The model under review builds one solid part; all positions refer to its coordinate system, in mm. A direction names the side the tool comes from. Round coordinates to 2 decimals unless told otherwise and drop trailing zeros. Loops run counter-clockwise (first coordinate to the right, second up) from the corner with the lowest first, then second, coordinate; pieces in that order, holes last. Notation, with made-up numbers: M 12.5,82.25 L 18.5,82.25 A18 ccw 18.5,105.25 Z; hole C 71,59 d8. An arc over 180 degrees is marked long. One line per question, with ' | ' between items.
from build123d import *

# Parameters (mm, degrees)
BOSS_EXTRUDE1_START      = 23
SKETCH1_W                = 6
SKETCH1_H                = 4
BOSS_EXTRUDE1_DEPTH      = 4.2
CUT_EXTRUDE1_DEPTH       = 24.280893454
CUT_EXTRUDE1_DEPTH_BACK  = 24.280893454
BOSS_EXTRUDE3_DEPTH      = 2
BOSS_EXTRUDE3_DEPTH_BACK = 2.5
FILLET2_R                = 1


with BuildPart() as part:
    # Sketch1 → Boss-Extrude1 (new body)
    with BuildSketch(Plane(origin=(0, 0, 0), x_dir=(0, 0, -1), z_dir=(1, 0, 0)).offset(BOSS_EXTRUDE1_START)):
        Rectangle(SKETCH1_W, SKETCH1_H)
    extrude(amount=-BOSS_EXTRUDE1_DEPTH)

    # Sketch2 → Cut-Extrude1 (cut, two sides)
    with BuildSketch(Plane(origin=(0, 0, 0), x_dir=(1, 0, 0), z_dir=(0, 1, 0))) as cut_extrude1_sk:
        with BuildLine():
            Line((22.422649731, 1), (11.5, 19.918584287))
            Line((11.5, 19.918584287), (23, 19.918584287))
            Line((23, 19.918584287), (23, -19.918584287))
            Line((23, -19.918584287), (11.5, -19.918584287))
            Line((11.5, -19.918584287), (22.422649731, -1))
            ThreePointArc((22.422649731, -1), (22.690598923, 0), (22.422649731, 1))
        make_face()
    extrude(amount=CUT_EXTRUDE1_DEPTH, mode=Mode.SUBTRACT)
    extrude(cut_extrude1_sk.sketch, amount=-CUT_EXTRUDE1_DEPTH_BACK, mode=Mode.SUBTRACT)

    # Sketch5 → Boss-Extrude3 (add, two sides)
    with BuildSketch(Plane(origin=(0, 0, 0), x_dir=(1, 0, 0), z_dir=(0, 1, 0))) as boss_extrude3_sk:
        Polygon((19.067949192, -3), (20.8, 0), (19.067949192, 3), (18.8, 3), (18.8, -3), align=None)
    extrude(amount=BOSS_EXTRUDE3_DEPTH)
    extrude(boss_extrude3_sk.sketch, amount=-BOSS_EXTRUDE3_DEPTH_BACK)

    # Fillet2
    fillet2_edges = [part.edges().sort_by_distance(p)[0] for p in [
        (20.167949192, -2, 3),
        (20.167949192, -2, -3),
        (20.033974596, 2, 3),
        (20.033974596, 2, -3),
    ]]
    fillet(fillet2_edges, radius=FILLET2_R)


solid = part.part
1) Add section C-C on z = 0.1. State the section outline as (x, y) points, then the cut area to 3 significant figures.
Output values:
outline: M 18.8,-2.5 L 20.74,-2.5 L 20.74,-2 L 22.69,-2 L 22.69,2 L 18.8,2 Z | area: 16.5 mm²
2) Add section B-B on x = 21. State the section outline as (y, z) points, then the cut area to 3 significant figures.
Output values:
outline: M -2,-2 A1 ccw -1,-3 L 1,-3 A1 ccw 2,-2 L 2,2 A1 ccw 1,3 L -1,3 A1 ccw -2,2 Z | area: 23.1 mm²
3) Machinability: for faces 1 (the cylindrical face through (20.437, -1.699, 2.715)), 2 (the cylindrical face through (20.437, -1.699, -2.715)), 3 (the flat face through (20, 0, 3)), which of the approach directions +Z, -Z, +X, -X, +Y, -Y give a long, thin tool a straight path to every point of the face, cutting with its end or side? Answer none if there is none.
Output values:
face 1: +Z, +X, -Y | face 2: -Z, +X, -Y | face 3: +Z, +X, -X, +Y, -Y
4) Add section D-D on x = 20.5. State the section outline as (y, z) points.
Output values:
outline: M -2.5,-0.52 L -2,-0.52 L -2,-2 A1 ccw -1,-3 L 1,-3 A1 ccw 2,-2 L 2,2 A1 ccw 1,3 L -1,3 A1 ccw -2,2 L -2,0.52 L -2.5,0.52 Z
5) Insertion check: P1, Ø1.5, axis at x = 22, z = 0, coming from the -Y side. The pin has a flat end and moves straight along its axis. Give the tip position at first contact, or say it passes through.
Output values:
P1: stops at y = -2
6) Add section A-A on y = 0.4. State the section outline as (x, z) points, then the cut area to 3 significant figures.
Output values:
outline: M 18.8,-3 L 21.27,-3 L 22.42,-1 A2 ccw 22.42,1 L 21.27,3 L 18.8,3 Z | area: 19.8 mm²
7) For line 1 (Y direction, x = 20.3, z = -1.75); line 2 (Z direction, x = 20.55, y = -2.15); line 3 (X direction, y = -2.1, z = 1), list the stretches that pass through material, from the lowest coordinate up.
Output values:
line 1: y = -2 to 2 | line 2: z = -0.43 to 0.43 | line 3: x = 18.8 to 20.22
